Part model, mm, in its own coordinate system. Face numbers are marked on the shaded views. A direction names the side the tool comes from. Coordinates: 2 decimals unless noted, no trailing zeros. Write each loop counter-clockwise with the first axis right and the second up, starting at its lowest first coordinate (ties: lowest second). Pieces come first, ordered by that corner, then holes. Notation, with made-up numbers: (46.5, 9) - (90.5, 9) arc R12 cw to (90.5, 28) - close; hole circle Ø2 at (11, 85.5). An arc over 180 degrees is marked (long way). Use a Markdown table: item, result.
```python
from build123d import *

# Parameters (mm, degrees)
F0_W           = 128.778
F0_H           = 125.476
F1_DEPTH       = 673.1
F2_W           = 88.9
F2_H           = 88.9
F3_DEPTH       = 508
F4_W           = 141.4779941578
F4_H           = 138.1759941578
F4_W_2         = 88.9
F4_H_2         = 88.9
F5_DEPTH       = 12.7
F6_W           = 141.4779941578
F6_H           = 138.1759941578
F6_W_2         = 128.778
F6_H_2         = 125.476
F7_DEPTH       = 6.35
F8_W           = 38.1
F8_H           = 38.1
F9_DEPTH       = 495.3
F10_W          = 139.7
F10_H          = 139.7
F10_W_2        = 127
F10_H_2        = 127
F11_DEPTH      = 6.35
F12_W          = 139.7
F12_H          = 139.7
F13_DEPTH      = 12.7
F14_W          = 50.8
F14_H          = 254
F15_DEPTH      = 19.05
F15_DEPTH_BACK = 107.95
F16_W          = 50.8
F16_H          = 254
F17_DEPTH      = 19.05
F17_DEPTH_BACK = 107.95
F18_W          = 139.7
F18_H          = 19.05
F19_DEPTH      = 133.35
F19_DEPTH_BACK = 6.35
F20_W          = 127
F20_H          = 127
F21_DEPTH      = 19.05


with BuildPart() as f1:
    # F0 (on Top) → F1 (new body)
    with BuildSketch(Plane.XY):
        Rectangle(F0_W, F0_H)
    extrude(amount=F1_DEPTH)

    # F2 (on face) → F3 (join)
    with BuildSketch(Plane.XY.offset(673.1)):
        Rectangle(F2_W, F2_H)
    extrude(amount=F3_DEPTH)

    # F4 (on face) → F5 (join)
    with BuildSketch(Plane.XY.offset(673.1)):
        Rectangle(F4_W, F4_H)
        Rectangle(F4_W_2, F4_H_2, mode=Mode.SUBTRACT)
    extrude(amount=F5_DEPTH)

    # F6 (on face) → F7 (join)
    with BuildSketch(Plane(origin=(0, 0, 673.1), x_dir=(1, 0, 0), z_dir=(0, 0, -1))):
        Rectangle(F6_W, F6_H)
        Rectangle(F6_W_2, F6_H_2, mode=Mode.SUBTRACT)
    extrude(amount=F7_DEPTH)

    # F8 (on face) → F9 (join)
    with BuildSketch(Plane.XY.offset(685.8)):
        with Locations((44.45, 44.45)):
            Rectangle(F8_W, F8_H)
        with Locations((44.45, -44.45)):
            Rectangle(F8_W, F8_H)
        with Locations((-44.45, -44.45)):
            Rectangle(F8_W, F8_H)
        with Locations((-44.45, 44.45)):
            Rectangle(F8_W, F8_H)
    extrude(amount=F9_DEPTH)

    # F10 (on face) → F11 (join)
    with BuildSketch(Plane.XY.offset(1181.1)):
        Rectangle(F10_W, F10_H)
        Rectangle(F10_W_2, F10_H_2, mode=Mode.SUBTRACT)
    extrude(amount=-F11_DEPTH)

    # F12 (on face) → F13 (join)
    with BuildSketch(Plane.XY.offset(1181.1)):
        Rectangle(F12_W, F12_H)
    extrude(amount=F13_DEPTH)

    # F14 (on face) → F15 (join, two sides)
    with BuildSketch(Plane.YZ.offset(44.45)) as f15_sk:
        with Locations((0, 1054.1)):
            Rectangle(F14_W, F14_H)
    extrude(amount=F15_DEPTH)
    extrude(f15_sk.sketch, amount=-F15_DEPTH_BACK)

    # F16 (on face) → F17 (join, two sides)
    with BuildSketch(Plane.XZ.offset(44.45)) as f17_sk:
        with Locations((0, 1054.1)):
            Rectangle(F16_W, F16_H)
    extrude(amount=F17_DEPTH)
    extrude(f17_sk.sketch, amount=-F17_DEPTH_BACK)

    # F18 (on face) → F19 (join, two sides)
    with BuildSketch(Plane.XZ.offset(63.5)) as f19_sk:
        with Locations((0, 917.575)):
            Rectangle(F18_W, F18_H)
    extrude(amount=-F19_DEPTH)
    extrude(f19_sk.sketch, amount=F19_DEPTH_BACK)

    # F20 (on face) → F21 (join)
    with BuildSketch(Plane.XY.offset(1193.8)):
        Rectangle(F20_W, F20_H)
    extrude(amount=F21_DEPTH)


solid = f1.part
```
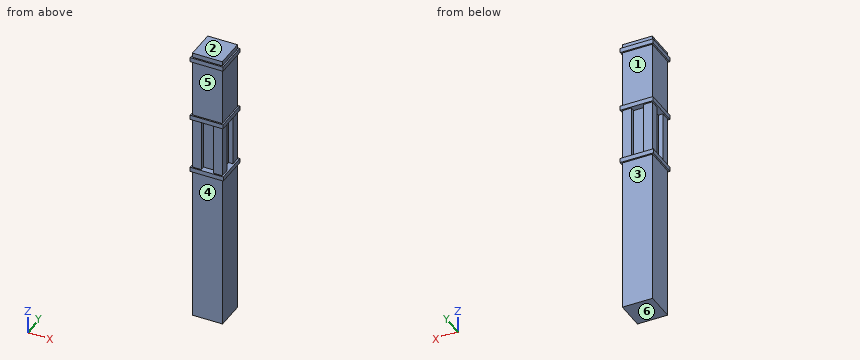
Item 1: Drill centre lines: probe 1 along Z at (x, y) = (-47, 14.5); probe 2 along Y at (x, z) = (-46, 900); probe 3 along X at (y, z) = (-29, 61.5). Where is each one in solid material? Low to high.
From the geometry:
| item | result |
|---|---|
| probe 1 | 0 to 685.8, 908.05 to 1212.85 |
| probe 2 | -63.5 to -25.4, 25.4 to 63.5 |
| probe 3 | -64.39 to 64.39 |
Item 2: Drop flat-ended pins along their axis: P1, Ø10, axis at x = -7, z = 849, coming from the +Y side; P2, Ø15, axis at y = -16.5, z = 1201, coming from the -X side; P3, Ø6, axis at x = -40, z = 261.5, coming from the +Y side. Give the stop position or say it passes through.
From the geometry:
| item | result |
|---|---|
| P1 | y = 44.45 |
| P2 | x = -69.85 |
| P3 | y = 62.74 |
Item 3: Band-saw the part on B-B, the plane z = 699.5. Give the cut face in (x, y), then the cut area to 3 significant figures.
From the geometry:
| item | result |
|---|---|
| outline | (-63.5, -63.5) - (-25.4, -63.5) - (-25.4, -44.45) - (25.4, -44.45) - (25.4, -63.5) - (63.5, -63.5) - (63.5, -25.4) - (44.45, -25.4) - (44.45, 25.4) - (63.5, 25.4) - (63.5, 63.5) - (25.4, 63.5) - (25.4, 44.45) - (-25.4, 44.45) - (-25.4, 63.5) - (-63.5, 63.5) - (-63.5, 25.4) - (-44.45, 25.4) - (-44.45, -25.4) - (-63.5, -25.4) - close |
| area | 12,300 mm^2 |
Item 4: Band-saw the part on C-C, the plane z = 130.5. Give the cut face in (x, y), then the cut area to 3 significant figures.
From the geometry:
| item | result |
|---|---|
| outline | (-64.39, -62.74) - (64.39, -62.74) - (64.39, 62.74) - (-64.39, 62.74) - close |
| area | 16,200 mm^2 |
Item 5: Which spindle directions (+Z, -Z, +X, -X, +Y, -Y) get a long thin tool onto all of the face, cutting with end or side? Do the marked faces 1, 2 and 3. Say none if no direction does.
From the geometry:
| item | result |
|---|---|
| face 1 | +X, -X, +Y |
| face 2 | +Z, +X, -X, +Y, -Y |
| face 3 | -Z, +X, -X, +Y |
Item 6: Band-saw the part on A-A, the plane y = 10. Give the cut face in (x, z).
From the geometry:
| item | result |
|---|---|
| outline | (-70.74, 666.75) - (-64.39, 666.75) - (-64.39, 0) - (64.39, 0) - (64.39, 666.75) - (70.74, 666.75) - (70.74, 685.8) - (44.45, 685.8) - (44.45, 908.05) - (69.85, 908.05) - (69.85, 927.1) - (63.5, 927.1) - (63.5, 1174.75) - (69.85, 1174.75) - (69.85, 1193.8) - (63.5, 1193.8) - (63.5, 1212.85) - (-63.5, 1212.85) - (-63.5, 1193.8) - (-69.85, 1193.8) - (-69.85, 1174.75) - (-63.5, 1174.75) - (-63.5, 927.1) - (-69.85, 927.1) - (-69.85, 908.05) - (-44.45, 908.05) - (-44.45, 685.8) - (-70.74, 685.8) - close |
Item 7: Band-saw the part on D-D, the plane z = 1007.5. Give the cut face in (x, y).
From the geometry:
| item | result |
|---|---|
| outline | (-63.5, -63.5) - (63.5, -63.5) - (63.5, 63.5) - (-63.5, 63.5) - close |
Item 8: Two-plate mould, pull along Z, no slides. Class the marked faces 4, 5 and 6: pulls with the +Z half, pulls with the -Z half, needs draft (parallel to the pull), parting line crosses it, or undercut.
From the geometry:
| item | result |
|---|---|
| face 4 | needs draft |
| face 5 | undercut |
| face 6 | pulls with the -Z half |
